```python
from build123d import *

# Parameters (mm, degrees)
F0_W     = 24.2
F0_H     = 17
F0_W_2   = 2
F0_H_2   = 14.65
F0_W_3   = 10.5
F0_H_3   = 1
F1_DEPTH = 2
F2_DEPTH = 20
F3_DEPTH = 5
F4_W     = 2
F4_H     = 12
F5_DEPTH = 20
F6_W     = 8
F6_H     = 5
F7_DEPTH = 25
F8_R     = 0.99999


# Not quite as in the source:
# - a fillet or chamfer is up to 0.001 mm smaller than in the source, because OpenCascade refuses the exact size


with BuildPart() as f1:
    # F0 (on Top) → F1 (new body)
    with BuildSketch(Plane.XY):
        Rectangle(F0_W, F0_H)
        Polygon((-10.1, 7.325), (-8.1, 7.325), (-8.1, 1), (2.4, 1), (2.4, 7.325), (4.4, 7.325), (4.4, -7.325), (2.4, -7.325), (2.4, -1), (-8.1, -1), (-8.1, -7.325), (-10.1, -7.325), align=None, mode=Mode.SUBTRACT)
        with Locations((10.1, 0)):
            Rectangle(F0_W_2, F0_H_2, mode=Mode.SUBTRACT)
        Polygon((-8.1, 1), (-8.1, 7.325), (-10.1, 7.325), (-10.1, -7.325), (-8.1, -7.325), (-8.1, -1), (-8.1, 0), align=None)
        Polygon((2.4, 7.325), (2.4, 1), (2.4, 0), (2.4, -1), (2.4, -7.325), (4.4, -7.325), (4.4, 7.325), align=None)
        with Locations((10.1, 0)):
            Rectangle(F0_W_2, F0_H_2)
        with Locations((-2.85, -0.5)):
            Rectangle(F0_W_3, F0_H_3)
        with Locations((-2.85, 0.5)):
            Rectangle(F0_W_3, F0_H_3)
    extrude(amount=-F1_DEPTH)

    # F0 (on Top) → F2 (join)
    with BuildSketch(Plane.XY):
        Polygon((-8.1, 1), (-8.1, 7.325), (-10.1, 7.325), (-10.1, -7.325), (-8.1, -7.325), (-8.1, -1), (-8.1, 0), align=None)
        with Locations((-2.85, 0.5)):
            Rectangle(F0_W_3, F0_H_3)
        Polygon((2.4, 7.325), (2.4, 1), (2.4, 0), (2.4, -1), (2.4, -7.325), (4.4, -7.325), (4.4, 7.325), align=None)
        with Locations((-2.85, -0.5)):
            Rectangle(F0_W_3, F0_H_3)
    extrude(amount=F2_DEPTH)

    # F0 (on Top) → F3 (join)
    with BuildSketch(Plane.XY):
        with Locations((10.1, 0)):
            Rectangle(F0_W_2, F0_H_2)
    extrude(amount=F3_DEPTH)

    # F4 (on face) → F5 (join)
    with BuildSketch(Plane(origin=(-10.1, 0, 0), x_dir=(0, -1, 0), z_dir=(-1, 0, 0))):
        with Locations((0, 12)):
            Rectangle(F4_W, F4_H)
    extrude(amount=F5_DEPTH)

    # F6 (on face) → F7 (cut)
    with BuildSketch(Plane(origin=(0, 1, 0), x_dir=(-1, 0, 0), z_dir=(0, 1, 0))):
        with Locations((22.1, 12)):
            Rectangle(F6_W, F6_H)
    extrude(amount=-F7_DEPTH, mode=Mode.SUBTRACT)

    # F8 (radius 1 in the source; OpenCascade refuses exactly that, so slightly less here)
    f8_edges = [f1.edges().sort_by_distance(p)[0] for p in [
        (-12.1, -8.5, -1),
        (-12.1, 8.5, -1),
        (12.1, -8.5, -1),
        (12.1, 8.5, -1),
        (11.1, -7.325, 2.5),
        (9.1, -7.325, 2.5),
        (11.1, 7.325, 2.5),
        (9.1, 7.325, 2.5),
        (2.4, -7.325, 10),
        (4.4, -7.325, 10),
        (-8.1, -7.325, 10),
        (-10.1, -7.325, 10),
        (-10.1, 7.325, 10),
        (-8.1, 7.325, 10),
        (2.4, 7.325, 10),
        (4.4, 7.325, 10),
        (-20.1, 1, 18),
        (-30.1, 1, 12),
        (-30.1, -1, 12),
        (-20.1, 1, 6),
        (-30.1, 0, 6),
        (-30.1, 0, 18),
        (-20.1, -1, 18),
        (-20.1, -1, 6),
        (-22.1, 1, 14.5),
        (-18.1, 1, 12),
        (-22.1, 1, 9.5),
        (-26.1, 1, 12),
        (-18.1, -1, 12),
        (-22.1, -1, 9.5),
        (-22.1, -1, 14.5),
        (-26.1, -1, 12),
    ]]
    fillet(f8_edges, radius=F8_R)


solid = f1.part
```
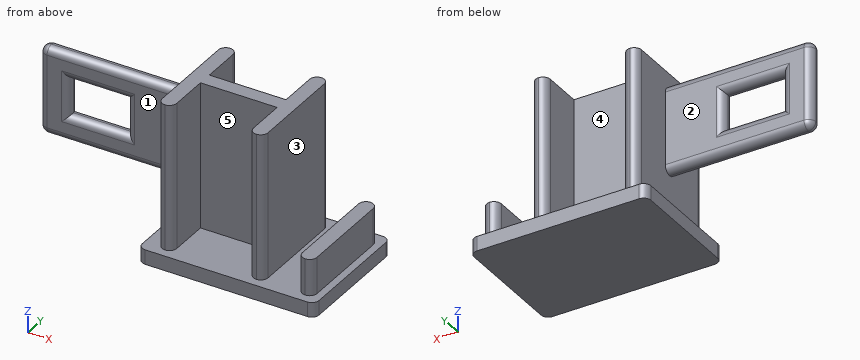
Check sheet for the modelled part. Datum: model origin and axes. Units: mm. Face numbers are marked on the shaded views. A direction names the side the tool comes from. Give positions to 0.01 mm unless a question says otherwise; leave off trailing zeros. Loops run counter-clockwise (first coordinate to the right, second up) from the corner with the lowest first, then second, coordinate; pieces in that order, holes last. Notation, with made-up numbers: (25.25, -28) - (84.25, -28) arc R15 cw to (84.25, -2) - close; hole circle Ø6 at (38.25, 19). An arc over 180 degrees is marked (long way). One line per question, with ' | ' between items. Start each with the question number.
1. Set-up check for the marked faces 1, 2, 3, 4 and 5: record each of +Z, -Z, +X, -X, +Y, -Y from which the full face is reachable in a straight line by a thin tool's end or side.
2. Gauge pin test, flat ends, axial feed: pin 1 Ø2 at (x, y) = (10, 2) entering from +Z; pin 2 Ø1.5 at (x, z) = (3.5, 17) entering from +Y (3 decimals); pin 3 Ø4 at (y, z) = (1.5, 12.5) entering from -X; pin 4 Ø4 at (x, y) = (-18, 4.5) entering from -Z. Record the tip position at first contact, or that the pin passes through.
3. Cross-section at D-D, the plane y = -4.75. Enter the section's corners in (x, z), plus the area to 3 significant figures.
4. Material ranges on line 1 along X through (y, z) = (3, 0.75); line 2 along X through (y, z) = (-3.75, 15); line 3 along Z through (x, y) = (-2, 6.5), recorded low to high. Write a range as [from, to].
Check result:
1) face 1: +Z, -X, -Y | face 2: +Z, -X, +Y | face 3: +Z, +Y, -Y | face 4: +Z, +Y | face 5: +Z, -Y
2) pin 1: stops at z = 5 | pin 2: stops at y = 7.325 | pin 3: stops at x = -30.1 | pin 4: passes through
3) outline: (-12.1, -2) - (12.1, -2) - (12.1, 0) - (11.1, 0) - (11.1, 5) - (9.1, 5) - (9.1, 0) - (4.4, 0) - (4.4, 20) - (2.4, 20) - (2.4, 0) - (-8.1, 0) - (-8.1, 20) - (-10.1, 20) - (-10.1, 0) - (-12.1, 0) - close | area: 138 mm2
4) line 1: x = [-10.1, -8.1], [2.4, 4.4], [9.1, 11.1] | line 2: x = [-10.1, -8.1], [2.4, 4.4] | line 3: z = [-2, 0]
